Check sheet for the modelled part. Datum: model origin and axes. Units: mm. A direction names the side the tool comes from. Coordinates: 2 decimals unless noted, no trailing zeros. Loops run counter-clockwise (first coordinate to the right, second up) from the corner with the lowest first, then second, coordinate; pieces in that order, holes last. Notation, with made-up numbers: (-12.75, 8) -> (45.25, 8) arc R15 ccw to (45.25, 36) -> close; hole circle Ø9 at (15, -9.75). An arc over 180 degrees is marked (long way). Use CSV: the item, a comma, the result in double quotes. Start each with the question number.
1. Sectioned sample at A-A, the plane z = -35.2. Count the separate pieces of the cut face and the enclosed holes in it, and give its area (3 significant figures).
2. Set-up check for faces 1 (the face through (-51, -19, -36)), 2 (the face through (-49.498, -24.245, -35.014)): record each of +Z, -Z, +X, -X, +Y, -Y from which the full face is reachable in a straight line by a thin tool's end or side.
3. Gauge pin test, flat ends, axial feed: pin 1 (1 mm diameter, centred on y = -21, z = -34.5, fed in from +X); pin 2 (3 mm diameter, centred on x = -52.5, y = -23, fed in from +Z); pin 3 (2 mm diameter, centred on x = -15.5, z = -37, fed in from +Y). Record the tip position at first contact, or that the pin passes through.
4. Thickness scan on L1, parallel to X at y = -23, z = -35.25; L2, parallel to X at y = -23, z = -37.5; L3, parallel to Y at x = 16.5, z = -36.4. Record the ranges inside material, lowest first.
5. Sectioned sample at B-B, the plane x = -50.5. Record the cut outline in (y, z), and give its area (3 significant figures).
6. Release check for a two-part mould opening along X. For faces 3 (the face through (20.14, -19.9, -35.97)), 4 (the face through (16, -24, -36)), 5 (the face through (-56.14, -19.9, -35.97)) record: pulls with the +X half, pulls with the -X half, needs draft (parallel to the pull), parting line crosses it, or undercut.
```python
from build123d import *

# Parameters (mm, degrees)
CYLINDER134_R     = 3.25
CYLINDER134_DEPTH = 3.5
CYLINDER136_R     = 0.6
CYLINDER136_DEPTH = 9.5
CYLINDER135_R     = 0.6
CYLINDER135_DEPTH = 9.5
CYLINDER133_R     = 3.25
CYLINDER133_DEPTH = 3.5
PAD012_DEPTH      = 4
FILLET076_R       = 3


with BuildPart() as zylinder134:
    # Cylinder134 → Cylinder134 (new body)
    with BuildSketch(Plane(origin=(-52.5, 23, -36), x_dir=(1, 0, 0), z_dir=(0, 0, 1))):
        Circle(CYLINDER134_R)
    extrude(amount=CYLINDER134_DEPTH)


with BuildPart() as zylinder136:
    # Cylinder136 → Cylinder136 (new body)
    with BuildSketch(Plane(origin=(16.5, 23, -39), x_dir=(1, 0, 0), z_dir=(0, 0, 1))):
        Circle(CYLINDER136_R)
    extrude(amount=CYLINDER136_DEPTH)


with BuildPart() as zylinder135:
    # Cylinder135 → Cylinder135 (new body)
    with BuildSketch(Plane(origin=(-52.5, 23, -39), x_dir=(1, 0, 0), z_dir=(0, 0, 1))):
        Circle(CYLINDER135_R)
    extrude(amount=CYLINDER135_DEPTH)


with BuildPart() as fusion087:
    # Cylinder133 → Cylinder133 (new body)
    with BuildSketch(Plane(origin=(16.5, 23, -36), x_dir=(1, 0, 0), z_dir=(0, 0, 1))):
        Circle(CYLINDER133_R)
    extrude(amount=CYLINDER133_DEPTH)

    # Fusion087: union Zylinder134, Zylinder136, Zylinder135
    add(zylinder134.part)
    add(zylinder136.part)
    add(zylinder135.part)


with BuildPart() as fillet076:
    # Sketch012 → Pad012 (new body)
    with BuildSketch(Plane.XY):
        with BuildLine():
            add(Edge.make_bspline(
                [(-48.5, 19), (-18, 24), (12.5, 19)],
                knots=[0, 0, 0, 1, 1, 1], degree=2))
            Line((-48.5, 19), (-57, 19))
            Line((-57, 19), (-57, 27))
            Line((-57, 27), (-48.5, 27))
            add(Edge.make_bspline(
                [(-48.5, 27), (-18, 22), (12.5, 27)],
                knots=[0, 0, 0, 1, 1, 1], degree=2))
            Line((12.5, 27), (21, 27))
            Line((21, 27), (21, 19))
            Line((21, 19), (12.5, 19))
        make_face()
    extrude(amount=PAD012_DEPTH)


with BuildPart() as fillet076_1:
    # Body003 placement: moved
    add(fillet076.part.moved(Location((0, 0, -38))))

    # Cut065: cut Fusion087
    add(fusion087.part, mode=Mode.SUBTRACT)

    # Fillet076
    fillet076_edges = [fillet076_1.edges().sort_by_distance(p)[0] for p in [
        (-57, 19, -36),
        (21, 19, -36),
        (-57, 27, -36),
        (21, 27, -36),
    ]]
    fillet(fillet076_edges, radius=FILLET076_R)


with BuildPart() as fillet076_2:
    # Fillet076 placement: moved
    add(fillet076_1.part.moved(Location((0, -46, 0))))


solid = fillet076_2.part
```
Completed:
1,separate pieces,"1"
1,enclosed holes,"2"
1,area,"347 mm²"
2,face 1,"+Z, -Z, +X, -X, +Y"
2,face 2,"+Z"
3,pin 1,"x = 20.96"
3,pin 2,"z = -36"
3,pin 3,"y = -21.47"
4,L1,"-57 to -55.75, -49.25 to 13.25, 19.75 to 21"
4,L2,"-57 to -53.1, -51.9 to 15.9, 17.1 to 21"
4,L3,"-27 to -23.6, -22.4 to -19"
5,outline,"(-27, -38) -> (-19, -38) -> (-19, -34) -> (-20.44, -34) -> (-20.44, -36) -> (-25.56, -36) -> (-25.56, -34) -> (-27, -34) -> close"
5,area,"21.8 mm²"
6,face 3,"pulls with the +X half"
6,face 4,"undercut"
6,face 5,"pulls with the -X half"
